Input: part model. Units: mm. Frame: model coordinates. A direction names the side the tool comes from. Round coordinates to 2 decimals unless told otherwise and drop trailing zeros. Loops run counter-clockwise (first coordinate to the right, second up) from the corner with the lowest first, then second, coordinate; pieces in that order, holes last.
(1) Cut plane A-A, the plane x = 0. Output: boundary loops of the cut face in (y, z), and give its area (3 significant figures).
(2) First-contact query: pin 1 Ø1.5 at (y, z) = (-11.5, -49.5) entering from +X; pin 2 Ø2 at (x, y) = (42, 3.5) entering from -Z; pin 3 Ø1.5 at (y, z) = (2.5, -69) entering from -X. Flat tips, straight axial feed; report the tip coordinate or a pass-through.
(3) Draft query along Z for faces 3 (the face through (-58.62, -0.35, -45.3)), 4 (the face through (-28, -15, -65)), 5 (the face through (0.09, -0.35, -72.05)), 6 (the face through (36.915, -13.496, -59.463)). Return one class per face: released by +Z, released by -Z, zero draft, split by the parting line, or undercut.
(4) Access query for faces 1 (the face through (52.1, 0.4, -40.3)), 2 (the face through (-36.772, -13.574, -59.385)). Directions: +Z, -Z, +X, -X, +Y, -Y. A direction counts if a zero-diameter tool reaches every point of the face in a straight line with its end or side. Return the directions, or none.
(5) Cut plane B-B, the plane y = 1.5. Output: boundary loops of the cut face in (x, z), and give its area (3 significant figures).
(6) Cut plane D-D, the plane x = 22. Output: boundary loops of the cut face in (y, z), and give its area (3 significant figures).
(7) Line query: line 1 (Z direction, x = 49.5, y = -2); line 2 (Y direction, x = 25, z = -65); line 3 (Z direction, x = -51, y = 23). Output: solid intervals per line, ascending.
(8) Cut plane C-C, the plane y = 20.5. Output: boundary loops of the cut face in (x, z), and give its area (3 significant figures).
from build123d import *

# Parameters (mm, degrees)
SKETCH_1_R          = 2.05
EXTRUDE_1_DEPTH     = 25
FILLET_2_R          = 3
CUT_EXTRUDE_1_DEPTH = 15
FILLET_3_R          = 5


with BuildPart() as part:
    # 草图1 → 凸台-拉伸1 (new, symmetric)
    with BuildSketch(Plane(origin=(0, 0, 0), x_dir=(1, 0, 0), z_dir=(0, 1, 0))):
        with BuildLine():
            Line((-59.897663254, 45.136126736), (-51.911308153, 39.117976505))
            ThreePointArc((-51.911308153, 39.117976505), (0, 65), (51.911308153, 39.117976505))
            Line((51.911308153, 39.117976505), (59.897663254, 45.136126736))
            ThreePointArc((59.897663254, 45.136126736), (0, 75), (-59.897663254, 45.136126736))
        make_face()
        with Locations(Location((-49.497474683, 49.497474683, 0), (0, 0, 270))):
            Circle(SKETCH_1_R, mode=Mode.SUBTRACT)
        with Locations(Location((0, 70, 0), (0, 0, 270))):
            Circle(SKETCH_1_R, mode=Mode.SUBTRACT)
        with Locations(Location((49.497474683, 49.497474683, 0), (0, 0, 270))):
            Circle(SKETCH_1_R, mode=Mode.SUBTRACT)
    extrude(amount=EXTRUDE_1_DEPTH, both=True)

    # 圆角2
    fillet_2_edges = [part.edges().sort_by_distance(p)[0] for p in [
        (-51.911308153, 0, -39.117976505),
        (-59.897663254, 0, -45.136126736),
        (59.897663254, 0, -45.136126736),
        (51.911308153, 0, -39.117976505),
    ]]
    fillet(fillet_2_edges, radius=FILLET_2_R)

    # 草图2 → 切除-拉伸1 (cut, symmetric)
    with BuildSketch(Plane(origin=(0, 0, 0), x_dir=(1, 0, 0), z_dir=(0, 1, 0))):
        with BuildLine():
            Line((-40.847927626, 62.900292596), (-35.401537276, 54.513586916))
            ThreePointArc((-35.401537276, 54.513586916), (-24.874423104, 60.052169613), (-13.514259903, 63.579594048))
            Line((-13.514259903, 63.579594048), (-15.593376811, 73.361070055))
            ThreePointArc((-15.593376811, 73.361070055), (-28.701257427, 69.290964938), (-40.847927626, 62.900292596))
        make_face()
        with BuildLine():
            ThreePointArc((13.514259903, 63.579594048), (24.874423104, 60.052169613), (35.401537276, 54.513586916))
            Line((35.401537276, 54.513586916), (40.847927626, 62.900292596))
            ThreePointArc((40.847927626, 62.900292596), (28.701257427, 69.290964938), (15.593376811, 73.361070055))
            Line((15.593376811, 73.361070055), (13.514259903, 63.579594048))
        make_face()
    extrude(amount=CUT_EXTRUDE_1_DEPTH, both=True, mode=Mode.SUBTRACT)

    # 圆角3
    fillet_3_edges = [part.edges().sort_by_distance(p)[0] for p in [
        (-38.124732451, 15, -58.706939756),
        (-14.553818357, -15, -68.470332051),
        (-38.124732451, -15, -58.706939756),
        (-14.553818357, 15, -68.470332051),
        (14.553818357, 15, -68.470332051),
        (38.124732451, -15, -58.706939756),
        (14.553818357, -15, -68.470332051),
        (38.124732451, 15, -58.706939756),
    ]]
    fillet(fillet_3_edges, radius=FILLET_3_R)


solid = part.part
Reported:
1. outline: (-25, -75) - (25, -75) - (25, -72.05) - (-25, -72.05) - close; (-25, -67.95) - (25, -67.95) - (25, -65) - (-25, -65) - close
1. area: 295 mm2
2. pin 1: stops at x = 57
2. pin 2: stops at z = -62.8
2. pin 3: stops at x = -14.83
3. face 3: split by the parting line
3. face 4: zero draft
3. face 5: undercut
3. face 6: released by -Z
4. face 1: +Z, +Y, -Y
4. face 2: -Z
5. outline: (-57.96, -47.59) arc R75 ccw to (-40.85, -62.9) - (-35.4, -54.51) arc R65 cw to (-50.13, -41.37) arc R3 ccw to (-54.25, -40.88) - (-57.45, -43.29) arc R3 ccw to start; (-15.59, -73.36) arc R75 ccw to (15.59, -73.36) - (13.51, -63.58) arc R65 cw to (-13.51, -63.58) - close; (35.4, -54.51) - (40.85, -62.9) arc R75 ccw to (57.96, -47.59) arc R3 ccw to (57.45, -43.29) - (54.25, -40.88) arc R3 ccw to (50.13, -41.37) arc R65 cw to start; hole circle Ø4.1 at (-49.5, -49.5); hole circle Ø4.1 at (0, -70); hole circle Ø4.1 at (49.5, -49.5)
5. area: 735 mm2
6. outline: (-25, -71.7) - (-15, -71.7) - (-15, -61.16) - (-25, -61.16) - close; (15, -71.7) - (25, -71.7) - (25, -61.16) - (15, -61.16) - close
6. area: 211 mm2
7. line 1: z = -56.34 to -51.55, -47.45 to -42.13
7. line 2: y = -25 to -15, 15 to 25
7. line 3: z = -54.99 to -50.89, -48.1 to -40.65
8. outline: (-57.96, -47.59) arc R75 ccw to (57.96, -47.59) arc R3 ccw to (57.45, -43.29) - (54.25, -40.88) arc R3 ccw to (50.13, -41.37) arc R65 cw to (-50.13, -41.37) arc R3 ccw to (-54.25, -40.88) - (-57.45, -43.29) arc R3 ccw to start; hole circle Ø4.1 at (-49.5, -49.5); hole circle Ø4.1 at (0, -70); hole circle Ø4.1 at (49.5, -49.5)
8. area: 1,250 mm2
